The listing builds one solid part. Answer for the finished solid, in the listing's coordinates (mm). Give positions to 0.01 mm unless a question says otherwise; leave off trailing zeros. Write each loop counter-clockwise with the first axis right and the second up, starting at its lowest first coordinate (ties: lowest second). Pieces come first, ordered by that corner, then holes. Notation, with made-up numbers: M 88.5,-27 L 147.5,-27 A17 cw 147.5,-14 Z; hole C 46.5,46.5 d10. An arc over 180 degrees is marked long. Return JSON: item names as keys, results as strings.
from build123d import *

# Parameters (mm, degrees)
BOSS_EXTRUDE1_DEPTH      = 1
BOSS_EXTRUDE1_DEPTH_BACK = 1
SKETCH1_R                = 1.25


with BuildPart() as part:
    # Sketch1 → Boss-Extrude1 (new, two sides: drawn at the far end of the back side and taken through both)
    with BuildSketch(Plane(origin=(0, 0, 0), x_dir=(0, 0, -1), z_dir=(1, 0, 0)).offset(-BOSS_EXTRUDE1_DEPTH_BACK)):
        with BuildLine():
            Line((-8.918483886, -23.220909654), (-8.616074, -22.433530013))
            ThreePointArc((-8.616074, -22.433530013), (-9.486095569, -18.843411487), (-13.151705182, -18.38603339))
            ThreePointArc((-13.151705182, -18.38603339), (-15.170840028, -18.712326304), (-16.985042177, -17.767845941))
            ThreePointArc((-16.985042177, -17.767845941), (-1.98e-07, 22.4), (16.985042454, -17.767845656))
            ThreePointArc((16.985042454, -17.767845656), (15.170840224, -18.712326272), (13.151705182, -18.38603339))
            ThreePointArc((13.151705182, -18.38603339), (9.486095569, -18.843411487), (8.616074, -22.433530013))
            Line((8.616074, -22.433530013), (8.918483886, -23.220909654))
            ThreePointArc((8.918483886, -23.220909654), (10.351464338, -24.65663681), (12.377500601, -24.557025041))
            ThreePointArc((12.377500601, -24.557025041), (-9.7e-08, 27.5), (-12.377500429, -24.557025128))
            ThreePointArc((-12.377500429, -24.557025128), (-10.351464248, -24.656636775), (-8.918483886, -23.220909654))
        make_face()
        with Locations((11.65, -21.26828625)):
            Circle(SKETCH1_R, mode=Mode.SUBTRACT)
        with Locations((-11.65, -21.26828625)):
            Circle(SKETCH1_R, mode=Mode.SUBTRACT)
    extrude(amount=BOSS_EXTRUDE1_DEPTH + BOSS_EXTRUDE1_DEPTH_BACK)


solid = part.part
Item 1: A cutting plane is placed at C-C, the plane x = 0.25. Count the separate pieces of the cut face and the enclosed holes in it, plus the area to 3 significant figures.
Geometry results:
{"separate pieces": "1", "enclosed holes": "2", "area": "595 mm2"}
Item 2: A cutting plane is placed at B-B, the plane z = -21. Write down the section's boundary in (x, y), plus the area to 3 significant figures.
Geometry results:
{"outline": "M -1,-17.76 L 1,-17.76 L 1,-12.21 L -1,-12.21 Z; M -1,9.66 L 1,9.66 L 1,17.76 L -1,17.76 Z", "area": "27.3 mm2"}
Item 3: A cutting plane is placed at D-D, the plane z = 11.65. Write down the section's boundary in (x, y).
Geometry results:
{"outline": "M -1,-24.79 L 1,-24.79 L 1,-22.52 L -1,-22.52 Z; M -1,-20.02 L 1,-20.02 L 1,-18.02 L -1,-18.02 Z; M -1,19.34 L 1,19.34 L 1,24.91 L -1,24.91 Z"}
Item 4: A cutting plane is placed at A-A, the plane y = 0. Write down the section's boundary in (x, z), plus the area to 3 significant figures.
Geometry results:
{"outline": "M -1,-27.5 L 1,-27.5 L 1,-23.64 L -1,-23.64 Z; M -1,23.64 L 1,23.64 L 1,27.5 L -1,27.5 Z", "area": "15.4 mm2"}
Item 5: Find the intervals of material crossed by line 1 (Z direction, x = -0.05, y = -0.5); line 2 (Y direction, x = 0.35, z = -11.5); line 3 (Y direction, x = -0.05, z = -11.65), in increasing order.
Geometry results:
{"line 1": "z = -27.5 to -23.66, 23.66 to 27.5", "line 2": "y = -24.81 to -22.51, -20.03 to -18.02, 19.42 to 24.98", "line 3": "y = -24.79 to -22.52, -20.02 to -18.02, 19.34 to 24.91"}
Item 6: Given pin 1 Ø1 at (x, y) = (0.5, 12) entering from +Z; pin 2 Ø6 at (y, z) = (-14.5, 6.5) entering from -X, each flat-ended and moving along its own axis, determine where each tip first touches the part or whether it passes through.
Geometry results:
{"pin 1": "stops at z = 24.98", "pin 2": "passes through"}
Item 7: Determine the mould class of faces 1 (the cylindrical face through (-0.01, -22.49, 11.92)), 2 (the flat face through (-1, 23, 2)), 3 (the cylindrical face through (-0.014, -24.667, 10.379)) for opening direction Y: +Y half, -Y half, draft (parallel to the pull), parting line (faces both ways), or undercut.
Geometry results:
{"face 1": "undercut", "face 2": "draft", "face 3": "-Y half"}
